CAD build for the part. Positions are in the model's coordinates, mm. Face numbers are marked on the shaded views. A direction names the side the tool comes from. Coordinates: 2 decimals unless noted, no trailing zeros. Order: outer loops, then holes, each group sorted by start corner. A loop starts at its lowest first (then second) coordinate and runs counter-clockwise, first axis right, second up. Notation, with made-up numbers: (-28.5, -9) - (-12.5, -9) arc R29 cw to (-12.5, 16) - close; hole circle Ø10 at (29.5, 34.5). An arc over 180 degrees is marked (long way). Return JSON: item names as keys, results as strings.
from build123d import *

# Parameters (mm, degrees)
SKETCH1_W           = 162
SKETCH1_H           = 140
BOSS_EXTRUDE2_DEPTH = 3
SKETCH2_W           = 162
SKETCH2_H           = 140
SKETCH2_W_2         = 156
SKETCH2_H_2         = 134
BOSS_EXTRUDE3_DEPTH = 47.5
SKETCH4_W           = 3
SKETCH4_H           = 134
BOSS_EXTRUDE4_DEPTH = 15
SKETCH5_R           = 1.575
SKETCH5_W           = 119
SKETCH5_H           = 20
CUT_EXTRUDE3_DEPTH  = 189.239873566
CUT_EXTRUDE4_REACH  = 176.503
SKETCH9_W           = 142
SKETCH9_H           = 5
CUT_EXTRUDE5_REACH  = 190.24
SKETCH10_W          = 30
SKETCH10_H          = 15


with BuildPart() as part:
    # Sketch1 → Boss-Extrude2 (new body)
    with BuildSketch(Plane(origin=(0, 0, 0), x_dir=(1, 0, 0), z_dir=(0, 1, 0))):
        Rectangle(SKETCH1_W, SKETCH1_H)
    extrude(amount=BOSS_EXTRUDE2_DEPTH)

    # Sketch2 → Boss-Extrude3 (add)
    with BuildSketch(Plane(origin=(0, 3, 0), x_dir=(1, 0, 0), z_dir=(0, 1, 0))):
        Rectangle(SKETCH2_W, SKETCH2_H)
        Rectangle(SKETCH2_W_2, SKETCH2_H_2, mode=Mode.SUBTRACT)
    extrude(amount=BOSS_EXTRUDE3_DEPTH)

    # Sketch4 → Boss-Extrude4 (add)
    with BuildSketch(Plane(origin=(0, 50.5, 0), x_dir=(1, 0, 0), z_dir=(0, 1, 0))):
        with Locations((-79.5, 0)):
            Rectangle(SKETCH4_W, SKETCH4_H)
        with Locations((79.5, 0)):
            Rectangle(SKETCH4_W, SKETCH4_H)
    extrude(amount=BOSS_EXTRUDE4_DEPTH)

    # Sketch5 → Cut-Extrude3 (cut, through all)
    with BuildSketch(Plane(origin=(81, 0, 0), x_dir=(0, 0, -1), z_dir=(1, 0, 0))):
        with Locations((59.5, 58)):
            Circle(SKETCH5_R)
        with Locations((-7.5, 55.5)):
            Rectangle(SKETCH5_W, SKETCH5_H)
    extrude(amount=-CUT_EXTRUDE3_DEPTH, mode=Mode.SUBTRACT)

    # Sketch9 → Cut-Extrude4 (cut, up to next)
    with BuildSketch(Plane.XY.offset(70), mode=Mode.PRIVATE) as cut_extrude4_sk1:
        with Locations((0, 48)):
            Rectangle(SKETCH9_W, SKETCH9_H)
    cut_extrude4_tool1 = extrude(cut_extrude4_sk1.sketch, amount=-CUT_EXTRUDE4_REACH, mode=Mode.PRIVATE) & part.part
    add(cut_extrude4_tool1.solids().sort_by_distance((0, 48, 70))[0], mode=Mode.SUBTRACT)

    # Sketch10 → Cut-Extrude5 (cut, up to next)
    with BuildSketch(Plane(origin=(81, 0, 0), x_dir=(0, 0, -1), z_dir=(1, 0, 0)), mode=Mode.PRIVATE) as cut_extrude5_sk1:
        with Locations((-39, 38)):
            Rectangle(SKETCH10_W, SKETCH10_H)
    cut_extrude5_tool1 = extrude(cut_extrude5_sk1.sketch, amount=-CUT_EXTRUDE5_REACH, mode=Mode.PRIVATE) & part.part
    add(cut_extrude5_tool1.solids().sort_by_distance((81, 38, 39))[0], mode=Mode.SUBTRACT)


solid = part.part
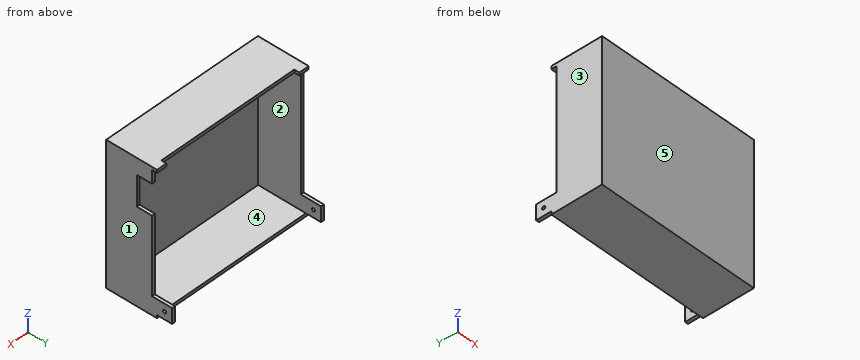
Item 1: Band-saw the part on B-B, the plane z = -54.5. List the corners of the cut face in (x, y), then the cut area to 3 significant figures.
Findings below:
{"outline": "(-81, 0) - (81, 0) - (81, 65.5) - (78, 65.5) - (78, 3) - (-78, 3) - (-78, 65.5) - (-81, 65.5) - close", "area": "861 mm²"}
Item 2: Band-saw the part on A-A, the plane y = 13. List the corners of the cut face in (x, z).
Findings below:
{"outline": "(-81, -70) - (81, -70) - (81, 70) - (-81, 70) - close; hole (-78, -67) - (78, -67) - (78, 67) - (-78, 67) - close"}
Item 3: Which spindle directions (+Z, -Z, +X, -X, +Y, -Y) get a long thin tool onto all of the face, cutting with end or side? Do the marked faces 4 and 5. Say none if no direction does.
Findings below:
{"face 4": "+Y", "face 5": "+Z, -Z, +X, -X, -Y"}
Item 4: Band-saw the part on C-C, the plane x = -15. List the corners of the cut face in (y, z), then the cut area to 3 significant figures.
Findings below:
{"outline": "(0, -70) - (50.5, -70) - (50.5, -67) - (3, -67) - (3, 67) - (45.5, 67) - (45.5, 70) - (0, 70) - close", "area": "690 mm²"}
Item 5: Band-saw the part on D-D, the plane y = 48. List the corners of the cut face in (x, z), then the cut area to 3 significant figures.
Findings below:
{"outline": "(-81, -70) - (81, -70) - (81, -52) - (78, -52) - (78, -67) - (-78, -67) - (-78, -52) - (-81, -52) - close; (-81, 67) - (-71, 67) - (-71, 70) - (-81, 70) - close; (71, 67) - (81, 67) - (81, 70) - (71, 70) - close", "area": "636 mm²"}
Item 6: Wall check: L1, parallel to Z at x = 25.5, y = 35; L2, parallel to X at y = 27, z = -58; L3, parallel to Y at x = -78.75, z = -59.5 (3 decimals). Give the ranges that are in metal, low to high. Write a range as [from, to].
Findings below:
{"L1": "z = [-70, -67], [67, 70]", "L2": "x = [-81, -78], [78, 81]", "L3": "y = [0, 56.425], [59.575, 65.5]"}
Item 7: Drop flat-ended pins along their axis: P1, Ø3.5, axis at x = 80, z = 63.5, coming from the +Y side; P2, Ø1.5, axis at x = -74, z = 68, coming from the +Y side; P3, Ø10, axis at x = -53, z = 15.5, coming from the +Y side. Give the stop position or say it passes through.
Findings below:
{"P1": "stops at y = 45.5", "P2": "stops at y = 50.5", "P3": "stops at y = 3"}
Item 8: Mould opens along X. For the marked faces 1, 2 and 3 say: released by +X, released by -X, zero draft, split by the parting line, or undercut.
Findings below:
{"face 1": "released by +X", "face 2": "undercut", "face 3": "released by -X"}
